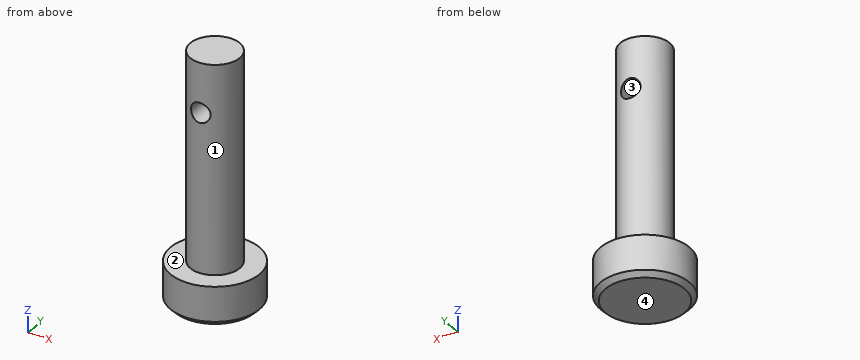
from build123d import *

# Parameters (mm, degrees)
MM_1_D         = 4
CHAMFER_1_SIZE = 1


with BuildPart() as part:
    # 草图1 → 旋转1 (revolve)
    with BuildSketch(Plane(origin=(0, 0, 0), x_dir=(0, 0, -1), z_dir=(1, 0, 0)), mode=Mode.PRIVATE) as revolve_1_sk:
        Polygon((0, 0), (0, 9), (-8, 9), (-8, 5), (-50, 5), (-50, 0), align=None)
    revolve(revolve_1_sk.sketch.rotate(Axis((0, 0, 50), (0, 0, -1)), 180), axis=Axis((0, 0, 50), (0, 0, -1)))

    # 大小mm 暗销孔1 (through all)
    with Locations(Plane(origin=(0, 5, 40), x_dir=(1, 0, 0), z_dir=(0, 1, 0))):
        with Locations((0, 0)):
            Hole(MM_1_D / 2)

    # 倒角1
    chamfer_1_edges = [part.edges().sort_by_distance(p)[0] for p in [
        (0, 9, 0),
    ]]
    chamfer(chamfer_1_edges, length=CHAMFER_1_SIZE)


solid = part.part
The model under review builds one solid part; all positions refer to its coordinate system, in mm. Face numbers are marked on the shaded views. Round coordinates to 2 decimals unless told otherwise and drop trailing zeros. Loops run counter-clockwise (first coordinate to the right, second up) from the corner with the lowest first, then second, coordinate; pieces in that order, holes last. Notation, with made-up numbers: M -19,-0.5 L -11,-0.5 A14 ccw -11,5.5 Z; hole C -24.75,47.5 d8. An arc over 180 degrees is marked long. Answer as CSV lines item,"result".
1. We need section A-A (x = 0). Give the boundary of the cut face in (y, z).
Outcome:
outline,"M -9,1 L -8,0 L 8,0 L 9,1 L 9,8 L 5,8 L 5,38 L -5,38 L -5,8 L -9,8 Z; M -5,42 L 5,42 L 5,50 L -5,50 Z"
2. Draft analysis for pull direction Z (two halves, no side actions). For the marked faces 1, 2, 3 and 4, state which applies: pulls with the +Z half, pulls with the -Z half, needs draft (parallel to the pull), parting line crosses it, or undercut.
Outcome:
face 1,"needs draft"
face 2,"pulls with the +Z half"
face 3,"undercut"
face 4,"pulls with the -Z half"
3. To check wall thickness, follow L1, parallel to Z at x = 0, y = -1.25; L2, parallel to Z at x = -3.5, y = 4.75; L3, parallel to Z at x = 1.5, y = -2.75. State the ranges of each line that lie inside material, in increasing order. Write a range as [from, to].
Outcome:
L1,"z = [0, 38], [42, 50]"
L2,"z = [0, 8]"
L3,"z = [0, 38.68], [41.32, 50]"
4. We need section D-D (z = 40). Give the boundary of the cut face in (x, y).
Outcome:
outline,"M -2,-4.58 L -2,4.58 A5 ccw Z; M 2,-4.58 A5 ccw 2,4.58 Z"
5. Insertion check: pin 1 Ø6 at (x, y) = (2.5, -6) entering from -Z; pin 2 Ø4 at (y, z) = (3, 16.5) entering from -X; pin 3 Ø3 at (x, z) = (-1.5, 17.5) entering from +Y; pin 4 Ø8 at (x, z) = (5.5, 31) entering from +Y. Each pin has a flat end and moves straight along its axis. Give the tip position at first contact, or say it passes through.
Outcome:
pin 1,"stops at z = 0"
pin 2,"stops at x = -4.9"
pin 3,"stops at y = 5"
pin 4,"stops at y = 4.77"
6. We need section C-C (z = 46). Give the boundary of the cut face in (x, y).
Outcome:
outline,"C 0,0 d10"
7. We need section B-B (y = 0). Give the boundary of the cut face in (x, z).
Outcome:
outline,"M -9,1 L -8,0 L 8,0 L 9,1 L 9,8 L 5,8 L 5,50 L -5,50 L -5,8 L -9,8 Z; hole C 0,40 d4"
